Autodesk Inventor part; units mm, degrees
ref_plane "YZ Plane" through (0, 0, 0) normal (1, 0, 0) x (0, 1, 0)
ref_plane "XZ Plane" through (0, 0, 0) normal (0, 1, 0) x (-1, 0, 0)
ref_plane "XY Plane" through (0, 0, 0) normal (0, 0, 1) x (1, 0, 0)
sketch "Sketch1" plane through (0, 0, 0) normal (0, 0, 1) x (1, 0, 0)
  circle A0 centre (0, 0) radius 16.8
  circle A1 centre (0, 0) radius 11.5
  circle A2 centre (0, 0) radius 17.8
  circle A3 centre (0, 0) radius 12.5
  dimension "d0" = 33.6
  dimension "d1" = 23
  dimension "d2" = 35.6
  dimension "d3" = 25
extrude "Extrusion1" add sketch "Sketch1" along normal blind 0.8 contours A3
extrude "Extrusion2" add sketch "Sketch1" along normal blind 3.2 contours A0
sketch "Sketch2" plane through (0, 0, 3.2) normal (0, 0, 1) x (1, 0, 0)
  circle A0 centre (0, 0) radius 17.8
  circle A1 centre (0, 0) radius 12.5
extrude "Extrusion3" add sketch "Sketch2" along normal blind 1.5
extrude "Extrusion5" add sketch "Sketch2" against normal blind 1
sketch "Sketch3" plane through (0, 0, 4.7) normal (0, 0, 1) x (1, 0, 0)
  line L0 (0.5, 4.5) -> (-0.5, 4.5)
  line L1 (-0.5, 4.5) -> (-0.5, 20.5)
  line L2 (-0.5, 20.5) -> (0.5, 20.5)
  line L3 (0.5, 20.5) -> (0.5, 4.5)
  circle A0 centre (0, 0) radius 12.5
  line L4 (0.5, 4.5) -> (-0.5, 20.5) construction
  line L5 (-0.5, 4.5) -> (0.5, 20.5) construction
  point P0 (0, 12.5)
  dimension "d10" = 1
  dimension "d11" = 16
extrude "Extrusion4" cut sketch "Sketch3" against normal blind 10 contours L0 L1 A0 L3 | A0 L1 L2 L3 picked at (0.0556, 7.1663)
properties part number "25to36mm-FilterAdapter"
Here's how the part is built. I have some questions about the finished solid (model axes, mm). A direction names the side the tool comes from. Coordinates: 2 decimals unless noted, no trailing zeros. Write each loop counter-clockwise with the first axis right and the second up, starting at its lowest first coordinate (ties: lowest second). Pieces come first, ordered by that corner, then holes.
1) If we section it at D-D (x = 0): List the corners of the cut face in (y, z) for me.
Filled in:
outline: (-17.8, 2.2) - (-16.8, 2.2) - (-16.8, 0) - (-11.5, 0) - (-11.5, 0.8) - (-12.5, 0.8) - (-12.5, 4.7) - (-17.8, 4.7) - close
2) I'm going to push a flat-ended pin straight in: pin 1 (1.4 mm diameter, centred on y = 15.5, z = 3, fed in from -X). Where does the tip first touch, or does it pass through?
Filled in:
pin 1: stops at x = -9.89
3) If we section it at C-C (z = 3.8): List the corners of the cut face in (x, y) for me, plus the area to 3 significant figures.
Filled in:
outline: (-0.5, 12.49) - (-0.5, 17.79) arc R17.8 ccw (long way) to (0.5, 17.79) - (0.5, 12.49) arc R12.5 cw (long way) to start
area: 499 mm2
4) Thinking about a two-plate mould opening in X: for faces 1 (the face through (11, -4, 0)), 2 (the face through (-0.5, 15, 2)), which applies, +X half, -X half, draft (parallel to the pull), parting line (faces both ways), or undercut?
Filled in:
face 1: draft
face 2: undercut
5) If we section it at B-B (x = 11): List the corners of the cut face in (y, z) for me, plus the area to 3 significant figures.
Filled in:
outline: (-13.99, 2.2) - (-12.7, 2.2) - (-12.7, 0) - (-3.35, 0) - (-3.35, 0.8) - (-5.94, 0.8) - (-5.94, 4.7) - (-13.99, 4.7) - close; (3.35, 0) - (12.7, 0) - (12.7, 2.2) - (13.99, 2.2) - (13.99, 4.7) - (5.94, 4.7) - (5.94, 0.8) - (3.35, 0.8) - close
area: 74.2 mm2
6) Which directions (+Z, -Z, +X, -X, +Y, -Y) give clear straight access to the entire face, cutting with the end or side of a thin tool? Please do faces 3 (the face through (0.5, 15, 2)), 4 (the face through (-6, -10, 0.8)), 5 (the face through (-11, -13, 2.2)), 6 (the face through (0.5, -11.49, 0.39)).
Filled in:
face 3: +Z, -Z, +Y
face 4: +Z
face 5: -Z
face 6: +Z, -Z
7) If I drill on line 1 (Y direction, x = 0, z = 2.9); line 2 (X direction, y = 0, z = 0.25); line 3 (Y direction, x = 0, z = 2), over which ranges is the centre line in solid material (lowest first)?
Filled in:
line 1: y = -17.8 to -12.5
line 2: x = -16.8 to -11.5, 11.5 to 16.8
line 3: y = -16.8 to -12.5
8) If we section it at A-A (y = 5): List the corners of the cut face in (x, z) for me.
Filled in:
outline: (-17.08, 2.2) - (-16.04, 2.2) - (-16.04, 0) - (-10.36, 0) - (-10.36, 0.8) - (-11.46, 0.8) - (-11.46, 4.7) - (-17.08, 4.7) - close; (10.36, 0) - (16.04, 0) - (16.04, 2.2) - (17.08, 2.2) - (17.08, 4.7) - (11.46, 4.7) - (11.46, 0.8) - (10.36, 0.8) - close
